Model file for the job. Use its own axes, mm. Face numbers are marked on the shaded views. A direction names the side the tool comes from. Coordinates: 2 decimals unless noted, no trailing zeros. Write each loop counter-clockwise with the first axis right and the second up, starting at its lowest first coordinate (ties: lowest second). Pieces come first, ordered by that corner, then holes.
Q1. Which spindle directions (+Z, -Z, +X, -X, +Y, -Y) get a long thin tool onto all of the face, cutting with end or side? Do the marked faces 4 and 5. Say none if no direction does.
Q2. Drill centre lines: probe 1 along Z at (x, y) = (0.5, 1); probe 2 along X at (y, z) = (-3.5, 1.25); probe 3 along X at (y, z) = (-3, 1.5). Where is each one in solid material? Low to high.
Q3. Pull direction X, two halves, no side cores. Call the marked faces 1, 2 and 3: released by +X, released by -X, zero draft, split by the parting line, or undercut.
Q4. Band-saw the part on A-A, the plane y = -3. Write the cut outline in (x, z), plus the area to 3 significant figures.
Q5. Pin check, flat tips, straight feed: P1, Ø4, axis at x = 0, z = 0, coming from the +Y side; P2, Ø2, axis at y = 2.5, z = 6.5, coming from the +X side; P3, Ø4, axis at x = -9, y = 0, coming from the -Z side; P4, Ø5, axis at y = 2.5, z = 8.5, coming from the +X side. Stop position of each tip, or through.
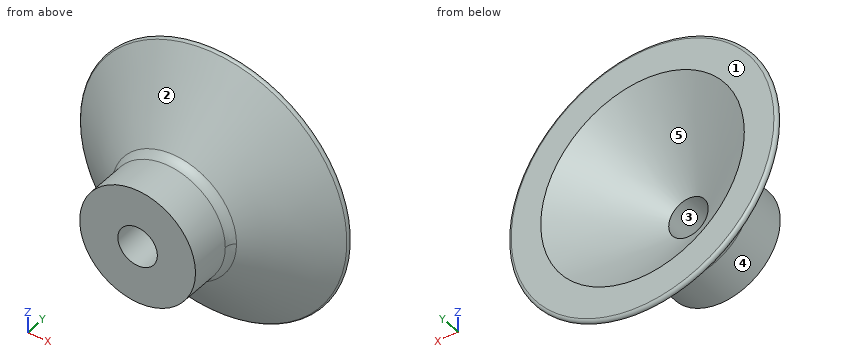
from build123d import *

# Parameters (mm, degrees)
SKETCH2_R           = 4.986862764
SKETCH2_R_2         = 1.7
BOSS_EXTRUDE1_DEPTH = 4
FILLET1_R           = 0.25
FILLET2_R           = 1


with BuildPart() as part:
    # Sketch1 → Revolve1 (revolve)
    with BuildSketch(Plane.XY):
        Polygon((-1.7, 0), (-4.986862764, 0), (-12.050794784, 5.416408), (-8.76393202, 5.416408), align=None)
    revolve(axis=Axis((0, 0, 0), (0, 1, 0)))

    # Sketch2 → Boss-Extrude1 (add)
    with BuildSketch(Plane.XZ):
        Circle(SKETCH2_R)
        Circle(SKETCH2_R_2, mode=Mode.SUBTRACT)
    extrude(amount=BOSS_EXTRUDE1_DEPTH)

    # Fillet1
    fillet1_edges = [part.edges().sort_by_distance(p)[0] for p in [
        (12.050794784, 5.416408, 0),
    ]]
    fillet(fillet1_edges, radius=FILLET1_R)

    # Fillet2
    fillet2_edges = [part.edges().sort_by_distance(p)[0] for p in [
        (0, 0, -4.986862764),
    ]]
    fillet(fillet2_edges, radius=FILLET2_R)


solid = part.part
Answer sheet:
1. face 4: -Y
1. face 5: +Y
2. probe 1: z = -6.27 to -2.96, 2.96 to 6.27
2. probe 2: x = -4.83 to -1.15, 1.15 to 4.83
2. probe 3: x = -4.76 to -0.8, 0.8 to 4.76
3. face 1: zero draft
3. face 2: split by the parting line
3. face 3: undercut
4. outline: circle Ø9.97 at (0, 0); hole circle Ø3.4 at (0, 0)
4. area: 69.0 mm2
5. P1: stops at y = 0.23
5. P2: stops at x = 7.21
5. P3: passes through
5. P4: stops at x = 8.37
